from build123d import *

# Parameters (mm, degrees)
F0_W     = 100
F0_H     = 50
F1_DEPTH = 20
F2_T     = -3
F3_R     = 3.5
F3_R_2   = 1
F3_W     = 10
F3_H     = 27
F4_DEPTH = 25
F6_DEPTH = 10


with BuildPart() as f1:
    # F0 (on Top) → F1 (new body)
    with BuildSketch(Plane.XY):
        Rectangle(F0_W, F0_H)
    extrude(amount=F1_DEPTH)

    # F2
    f2_openings = [f1.faces().sort_by_distance(p)[0] for p in [
        (0, 0, 0),
    ]]
    offset(amount=F2_T, openings=f2_openings)

    # F3 (on face) → F4 (cut)
    with BuildSketch(Plane.XY.offset(20)):
        Circle(F3_R)
        with Locations((0, 7)):
            Circle(F3_R_2)
        with Locations((-6.0621778265, 3.5)):
            Circle(F3_R_2)
        with Locations((-6.0621778265, -3.5)):
            Circle(F3_R_2)
        with Locations((0, -7)):
            Circle(F3_R_2)
        with Locations((6.0621778265, -3.5)):
            Circle(F3_R_2)
        with Locations((6.0621778265, 3.5)):
            Circle(F3_R_2)
        with Locations((-28, 0)):
            Rectangle(F3_W, F3_H)
        with Locations((28, 0)):
            Rectangle(F3_W, F3_H)
    extrude(amount=-F4_DEPTH, mode=Mode.SUBTRACT)

    # F5 (on Front) → F6 (join, symmetric)
    with BuildSketch(Plane.XZ):
        with BuildLine():
            Line((33, 20), (50, 20))
            Line((50, 20), (50, 23))
            add(Edge.make_bspline(
                [(33, 21), (36.8661454102, 21.3032203159), (43.6623686797, 21.8362455253), (48.0907692486, 22.6494154176), (50, 23)],
                knots=[0, 0, 0, 0, 0.5688667451, 1, 1, 1, 1], degree=3))
            Line((33, 21), (33, 20))
        make_face()
        with BuildLine():
            Line((-50, 23), (-50, 20))
            Line((-50, 20), (-33, 20))
            add(Edge.make_bspline(
                [(-50, 23), (-47.7477722772, 22.3250847317), (-43.9802378635, 20.1526522743), (-36.3079621025, 20.101446954), (-33, 20)],
                knots=[0, 0, 0, 0, 0.4421409573, 1, 1, 1, 1], degree=3))
        make_face()
    extrude(amount=F6_DEPTH, both=True)


solid = f1.part
Verification items for the finished model (mm, model axes). A direction names the side the tool comes from. Coordinates: 2 decimals unless noted, no trailing zeros. Order: outer loops, then holes, each group sorted by start corner. A loop starts at its lowest first (then second) coordinate and runs counter-clockwise, first axis right, second up. Notation, with made-up numbers: M -3.5,62.5 L 19.5,62.5 A13 cw 19.5,87.5 Z; hole C -40,40 d5. An arc over 180 degrees is marked long. One line per item, written item: value. Start each with the question number.
Item 1: Sectioned sample at A-A on x = 0. Record the cut outline in (y, z).
Item 2: Sectioned sample at C-C on x = -31. Record the cut outline in (y, z).
Item 3: Sectioned sample at D-D on y = -21. Record the cut outline in (x, z), then the cut area to 3 significant figures.
Item 4: Depth check by flat-ended pin: P1, Ø2.5, axis at x = -40.5, z = 21.5, coming from the -Y side; P2, Ø3, axis at x = -7.5, y = -2, coming from the -Z side; P3, Ø0.9, axis at x = 45.5, z = 22, coming from the +Y side; P4, Ø0.9, axis at x = -40, z = 21, coming from the +Y side. Enter the tip coordinate at first touch or a pass-through.
Item 5: Thickness scan on probe 1 along Y at (x, z) = (-13, 15.5); probe 2 along Y at (x, z) = (0, 18.4); probe 3 along X at (y, z) = (14, 6.25). Record the ranges inside material, lowest first.
Item 6: Access from +Z, -Z, +X, -X, +Y, -Y to the whole of each face (thin tool, end or side, straight path). Record for faces 1 (the flat face through (28, -13.5, 19)), 2 (the flat face through (43, -10, 21)), 3 (the flat face through (43, 10, 21)).
Item 7: Sectioned sample at B-B on z = 18.5. Give the number of separate pieces and of enclosed holes in the cut face, then the cut area to 3 significant figures.
Calculated:
1. outline: M -25,0 L -22,0 L -22,17 L -8,17 L -8,20 L -25,20 Z; M -6,17 L -3.5,17 L -3.5,20 L -6,20 Z; M 3.5,17 L 6,17 L 6,20 L 3.5,20 Z; M 8,17 L 22,17 L 22,0 L 25,0 L 25,20 L 8,20 Z
2. outline: M -25,0 L -22,0 L -22,17 L -13.5,17 L -13.5,20 L -25,20 Z; M 13.5,17 L 22,17 L 22,0 L 25,0 L 25,20 L 13.5,20 Z
3. outline: M -50,0 L -47,0 L -47,17 L 47,17 L 47,0 L 50,0 L 50,20 L -50,20 Z
3. area: 402 mm^2
4. P1: y = -10
4. P2: z = 17
4. P3: y = 10
4. P4: through
5. probe 1: -25 to -22, 22 to 25
5. probe 2: -25 to -8, -6 to -3.5, 3.5 to 6, 8 to 25
5. probe 3: -50 to -47, 47 to 50
6. face 1: +Z, -Z
6. face 2: +Z, +X, -X, -Y
6. face 3: +Z, +X, -X, +Y
7. separate pieces: 1
7. enclosed holes: 9
7. area: 4,400 mm^2
